```python
from build123d import *

# Parameters (mm, degrees)
SKETCH7_W           = 34.5
SKETCH7_H           = 10
BOSS_EXTRUDE3_DEPTH = 20
CUT_EXTRUDE9_DEPTH  = 26
SKETCH9_R           = 5
CUT_EXTRUDE10_DEPTH = 26


with BuildPart() as part:
    # Sketch7 → Boss-Extrude3 (new body)
    with BuildSketch(Plane(origin=(0, 0, 0), x_dir=(1, 0, 0), z_dir=(0, 1, 0))):
        with Locations((17.25, 0)):
            Rectangle(SKETCH7_W, SKETCH7_H)
    extrude(amount=BOSS_EXTRUDE3_DEPTH)

    # Sketch8 → Cut-Extrude9 (cut)
    with BuildSketch(Plane(origin=(0, 0, -5), x_dir=(-1, 0, 0), z_dir=(0, 0, -1))):
        with BuildLine():
            Line((-10, 20), (6.269101311, 20))
            Line((6.269101311, 20), (6.269101311, 0))
            Line((6.269101311, 0), (-10, 0))
            ThreePointArc((-10, 0), (0, 10), (-10, 20))
        make_face()
    extrude(amount=-CUT_EXTRUDE9_DEPTH, mode=Mode.SUBTRACT)

    # Sketch9 → Cut-Extrude10 (cut)
    with BuildSketch(Plane(origin=(0, 0, -5), x_dir=(-1, 0, 0), z_dir=(0, 0, -1))):
        with Locations((-10, 10)):
            Circle(SKETCH9_R)
    extrude(amount=-CUT_EXTRUDE10_DEPTH, mode=Mode.SUBTRACT)


solid = part.part
```
Could you check a few things on this model? Use its own coordinates, in mm. Coordinates: 2 decimals unless noted, no trailing zeros. Loops run counter-clockwise (first coordinate to the right, second up) from the corner with the lowest first, then second, coordinate; pieces in that order, holes last.
1) Will these pins go through, and if not, where does the flat tip stop? pin 1 Ø9 at (x, y) = (10, 10) entering from -Z; pin 2 Ø2 at (y, z) = (14, -2) entering from -X.
Reported:
pin 1: passes through
pin 2: stops at x = 0.46
2) Imagine slicing it at D-D (y = 15.75). List the corners of the cut face in (x, z) for me.
Reported:
outline: (1.82, -5) - (34.5, -5) - (34.5, 5) - (1.82, 5) - close
3) Imagine slicing it at C-C (z = 0). List the corners of the cut face in (x, y) for me.
Reported:
outline: (10, 0) - (34.5, 0) - (34.5, 20) - (10, 20) arc R10 ccw to start; hole circle Ø10 at (10, 10)
4) Imagine slicing it at A-A (y = 10). List the corners of the cut face in (x, z) for me, and give its area (3 significant figures).
Reported:
outline: (0, -5) - (5, -5) - (5, 5) - (0, 5) - close; (15, -5) - (34.5, -5) - (34.5, 5) - (15, 5) - close
area: 245 mm2
5) Please list where these lines run through material, in increasing order: line 1 along Y through (x, z) = (10, -1.25); line 2 along X through (y, z) = (9.75, -3); line 3 along Y through (x, z) = (13, 1.5).
Reported:
line 1: y = 0 to 5, 15 to 20
line 2: x = 0 to 5.01, 14.99 to 34.5
line 3: y = 0 to 6, 14 to 20
6) Thinking about a two-plate mould opening in X: for faces 1 (the face through (34.5, 10, 0)), 2 (the face through (0, 10, 0)), 3 (the face through (5.23, 11.5, -0.07)), 4 (the face through (22, 0, 0)), which applies, released by +X, released by -X, zero draft, split by the parting line, or undercut?
Reported:
face 1: released by +X
face 2: released by -X
face 3: undercut
face 4: zero draft
7) Imagine slicing it at B-B (x = 9). List the corners of the cut face in (y, z) for me.
Reported:
outline: (0.05, -5) - (5.1, -5) - (5.1, 5) - (0.05, 5) - close; (14.9, -5) - (19.95, -5) - (19.95, 5) - (14.9, 5) - close
